The model under review builds one solid part; all positions refer to its coordinate system, in mm. Face numbers are marked on the shaded views. Coordinates: 2 decimals unless noted, no trailing zeros. Write each loop counter-clockwise with the first axis right and the second up, starting at its lowest first coordinate (ties: lowest second). Pieces come first, ordered by that corner, then holes.
1) Add section D-D, the plane z = -18. State the section outline as (x, y) points.
2) Add section A-A, the plane x = 0. State the section outline as (y, z) points (3 decimals).
3) For P1, Ø4, axis at x = 14, y = -22.5, coming from the +Z side; P2, Ø1.5, axis at x = 14, y = -20.5, coming from the -Z side; P3, Ø8, axis at x = 18, y = -26, coming from the +Z side, all flat-tipped, find the tip position at first contact; note any pin that passes through.
4) Add section C-C, the plane y = -5. State the section outline as (x, z) points (3 decimals), then the cut area to 3 significant figures.
5) For line 1 (Z direction, x = 0, y = -16) (3 decimals); line 2 (Y direction, x = -7, z = 21); line 3 (X direction, y = -13, z = 0.5), list the stretches that pass through material, from the lowest coordinate up.
6) Mouldability with a two-part tool opening along Z and no side actions: class the marked faces 1, 2, 3 and 4 as released by +Z, released by -Z, zero draft, split by the parting line, or undercut.
7) Add section B-B, the plane z = 3. State the section outline as (x, y) points.
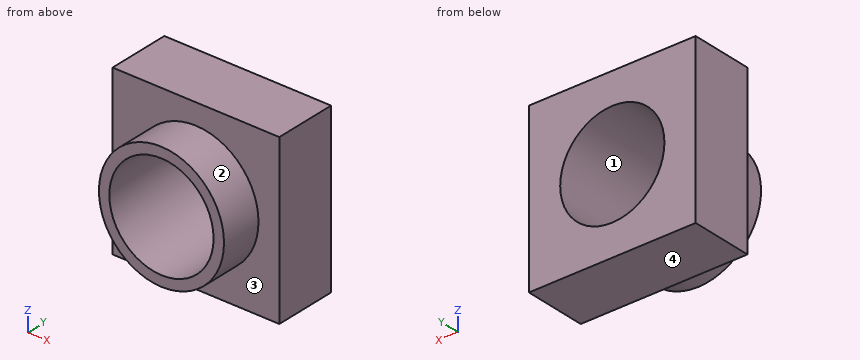
from build123d import *

# Parameters (mm, degrees)
F0_W     = 50.8
F0_H     = 50.8
F1_DEPTH = 19.05
F2_R     = 19.05
F3_DEPTH = 12.7
F4_R     = 15.875
F5_DEPTH = 50.292


with BuildPart() as f1:
    # F0 (on Front) → F1 (new body)
    with BuildSketch(Plane.XZ):
        Rectangle(F0_W, F0_H)
    extrude(amount=F1_DEPTH)

    # F2 (on face) → F3 (join)
    with BuildSketch(Plane.XZ.offset(19.05)):
        Circle(F2_R)
    extrude(amount=F3_DEPTH)

    # F4 (on face) → F5 (cut)
    with BuildSketch(Plane.XZ.offset(31.75)):
        Circle(F4_R)
    extrude(amount=-F5_DEPTH, mode=Mode.SUBTRACT)


solid = f1.part
Geometry results:
1. outline: (-25.4, -19.05) - (-6.24, -19.05) - (-6.24, -31.75) - (6.24, -31.75) - (6.24, -19.05) - (25.4, -19.05) - (25.4, 0) - (-25.4, 0) - close
2. outline: (-31.75, -19.05) - (-19.05, -19.05) - (-19.05, -25.4) - (0, -25.4) - (0, -15.875) - (-31.75, -15.875) - close; (-31.75, 15.875) - (0, 15.875) - (0, 25.4) - (-19.05, 25.4) - (-19.05, 19.05) - (-31.75, 19.05) - close
3. P1: stops at z = 14.8
3. P2: stops at z = -13.69
3. P3: stops at z = 12.92
4. outline: (-25.4, -25.4) - (25.4, -25.4) - (25.4, 25.4) - (-25.4, 25.4) - close; hole circle Ø31.75 at (0, 0)
4. area: 1,790 mm2
5. line 1: z = -25.4 to -15.875, 15.875 to 25.4
5. line 2: y = -19.05 to 0
5. line 3: x = -25.4 to -15.87, 15.87 to 25.4
6. face 1: undercut
6. face 2: split by the parting line
6. face 3: zero draft
6. face 4: released by -Z
7. outline: (-25.4, -19.05) - (-18.81, -19.05) - (-18.81, -31.75) - (-15.59, -31.75) - (-15.59, 0) - (-25.4, 0) - close; (15.59, -31.75) - (18.81, -31.75) - (18.81, -19.05) - (25.4, -19.05) - (25.4, 0) - (15.59, 0) - close
